Source: CAD feature listing. Evaluate the final solid. Frame: model axes, mm. A direction names the side the tool comes from. Give positions to 0.01 mm unless a question says otherwise; leave off trailing zeros. Loops run counter-clockwise (first coordinate to the right, second up) from the corner with the lowest first, then second, coordinate; pieces in that order, holes last. Notation, with made-up numbers: (81, 16) - (101, 16) arc R16 cw to (101, 31) - close; hole circle Ø4 at (-28.75, -14). An arc over 180 degrees is marked (long way). Write each question's results on one line, items separated by ' | '. Start each with the question number.
(1) Cut plane D-D on y = 0.25. Return the cut outline in (x, z).
(2) Cut plane A-A on x = 1.25. Return the cut outline in (y, z) (3 decimals), then the cut area to 3 significant figures.
(3) Cut plane B-B on y = -1. Return the cut outline in (x, z), then the cut area to 3 significant figures.
(4) Pull-direction query (X, two-part tool) for faces 4 (the cylindrical face through (1.126, -0.809, -0.507)), 5 (the flat face through (0, 0, 5)); classes: pulls with the +X half, pulls with the -X half, needs draft (parallel to the pull), parting line crosses it, or undercut.
(5) Contact query for flat-ended pins moving along their axis: pin 1 (1 mm diameter, centred on x = 0.5, z = 4, fed in from -Y); pin 2 (2 mm diameter, centred on x = 1.73, y = -1, fed in from -Z); pin 3 (4 mm diameter, centred on y = 3, z = 0.5, fed in from +X); pin 4 (1 mm diameter, centred on y = 2.5, z = 2.5, fed in from +X). Output: stop coordinate, or through.
(6) Reachability of faces 1 (the flat face through (-1.59, 2, 2)), 2 (the flat face through (0, 0, -1)), 3 (the cylindrical face through (-1.098, -0.972, -0.507)) from +Z, -Z, +X, -X, +Y, -Y: full face, straight path, thin tool, end or side. Return the list, or none.
(7) Cut plane C-C on z = 4. Return the cut outline in (x, y) (3 decimals).
(8) Material intervals for line 1 along Y through (x, z) = (0, 4.5) (3 decimals); line 2 along Y through (x, z) = (1, 3.25) (3 decimals); line 3 along X through (y, z) = (0.5, 0.75), sorted ascending. Write a range as [from, to].
from build123d import *

# Parameters (mm, degrees)
SKETCH1_R           = 4
SKETCH1_W           = 3.18
SKETCH1_H           = 2.03
BOSS_EXTRUDE1_DEPTH = 5
BOSS_EXTRUDE3_START = 1
SKETCH4_R           = 4
SKETCH4_R_2         = 0.635
BOSS_EXTRUDE3_DEPTH = 1
SKETCH2_R           = 0.725
BOSS_EXTRUDE2_DEPTH = 0.725
FILLET2_R           = 0.725
SKETCH3_R           = 0.75
CUT_EXTRUDE2_DEPTH  = 0.75
FILLET3_R           = 0.75


with BuildPart() as part:
    # Sketch1 → Boss-Extrude1 (new body)
    with BuildSketch(Plane.XY):
        Circle(SKETCH1_R)
        Polygon((3.406066592, -0.130519608), (1.648035023, 0.884480392), (0.058035023, -1.869480392), (1.816066592, -2.884480392), align=None, mode=Mode.SUBTRACT)
        with Locations((0, 2)):
            Rectangle(SKETCH1_W, SKETCH1_H, mode=Mode.SUBTRACT)
        Polygon((-1.740313417, -2.765688741), (-0.198788198, -1.875688741), (-1.723788198, 0.765688741), (-3.265313417, -0.124311259), align=None, mode=Mode.SUBTRACT)
    extrude(amount=BOSS_EXTRUDE1_DEPTH)

    # Sketch4 → Boss-Extrude3 (add)
    with BuildSketch(Plane(origin=(0, 0, 0), x_dir=(-1, 0, 0), z_dir=(0, 0, -1)).offset(BOSS_EXTRUDE3_START)):
        Circle(SKETCH4_R)
        with Locations((0, 2)):
            Circle(SKETCH4_R_2, mode=Mode.SUBTRACT)
        with Locations((1.732050808, -1)):
            Circle(SKETCH4_R_2, mode=Mode.SUBTRACT)
        with Locations((-1.732050808, -1)):
            Circle(SKETCH4_R_2, mode=Mode.SUBTRACT)
    extrude(amount=-BOSS_EXTRUDE3_DEPTH)

    # Sketch2 → Boss-Extrude2 (add)
    with BuildSketch(Plane(origin=(0, 0, -1), x_dir=(-1, 0, 0), z_dir=(0, 0, -1))):
        with Locations((0, -3)):
            Circle(SKETCH2_R)
        with Locations((-2.598076211, 1.5)):
            Circle(SKETCH2_R)
        with Locations((2.598076211, 1.5)):
            Circle(SKETCH2_R)
    extrude(amount=BOSS_EXTRUDE2_DEPTH)

    # Fillet2
    fillet2_edges = [part.edges().sort_by_distance(p)[0] for p in [
        (0.725, -3, -1.725),
        (3.323076211, 1.5, -1.725),
        (-1.873076211, 1.5, -1.725),
    ]]
    fillet(fillet2_edges, radius=FILLET2_R - 0.0001)  # a hair under: the kernel refuses the full size

    # Sketch3 → Cut-Extrude2 (cut)
    with BuildSketch(Plane.XY.offset(5)):
        with Locations((0, -3)):
            Circle(SKETCH3_R)
        with Locations((-2.598076211, 1.5)):
            Circle(SKETCH3_R)
        with Locations((2.598076211, 1.5)):
            Circle(SKETCH3_R)
    extrude(amount=-CUT_EXTRUDE2_DEPTH, mode=Mode.SUBTRACT)

    # Fillet3
    fillet3_edges = [part.edges().sort_by_distance(p)[0] for p in [
        (-0.75, -3, 4.25),
        (-3.348076211, 1.5, 4.25),
        (1.848076211, 1.5, 4.25),
    ]]
    fillet(fillet3_edges, radius=FILLET3_R - 0.0001)  # a hair under: the kernel refuses the full size


solid = part.part
Ans:
1) outline: (-3.99, -1) - (3.99, -1) - (3.99, 5) - (2.75, 5) - (2.75, 0) - (1.28, 0) - (1.28, 5) - (-1.43, 5) - (-1.43, 0) - (-2.62, 0) - (-2.62, 5) - (-3.99, 5) - close
2) outline: (-3.8, -1) - (-1.413, -1) - (-1.413, 0) - (-2.558, 0) - (-2.558, 5) - (-3.8, 5) - close; (-0.587, -1) - (3.8, -1) - (3.8, 5) - (3.015, 5) - (3.015, 0) - (0.985, 0) - (0.985, 5) - (0.195, 5) - (0.195, 0) - (-0.587, 0) - close | area: 20.9 mm^2
3) outline: (-3.87, -1) - (-2.37, -1) - (-2.37, 0) - (-2.76, 0) - (-2.76, 5) - (-3.87, 5) - close; (-1.1, -1) - (1.1, -1) - (1.1, 0) - (0.56, 0) - (0.56, 5) - (-0.7, 5) - (-0.7, 0) - (-1.1, 0) - close; (2.37, -1) - (3.87, -1) - (3.87, 5) - (2.9, 5) - (2.9, 0) - (2.37, 0) - close | area: 21.9 mm^2
4) face 4: undercut | face 5: needs draft
5) pin 1: y = -4 | pin 2: z = -1 | pin 3: x = 3.87 | pin 4: x = 3.46
6) face 1: +Z | face 2: -Z | face 3: +Z, -Z
7) outline: circle Ø8 at (0, 0); hole (-3.265, -0.124) - (-1.74, -2.766) - (-0.199, -1.876) - (-1.724, 0.766) - close; hole (-1.59, 0.985) - (1.59, 0.985) - (1.59, 3.015) - (-1.59, 3.015) - close; hole (0.058, -1.869) - (1.816, -2.884) - (3.406, -0.131) - (1.648, 0.884) - close
8) line 1: [-4, -3.559], [-2.441, 0.985], [3.015, 4] | line 2: [-3.873, -2.413], [-0.238, 0.985], [3.015, 3.873] | line 3: [-3.97, -2.18], [-1.57, 1.43], [2.31, 3.97]
